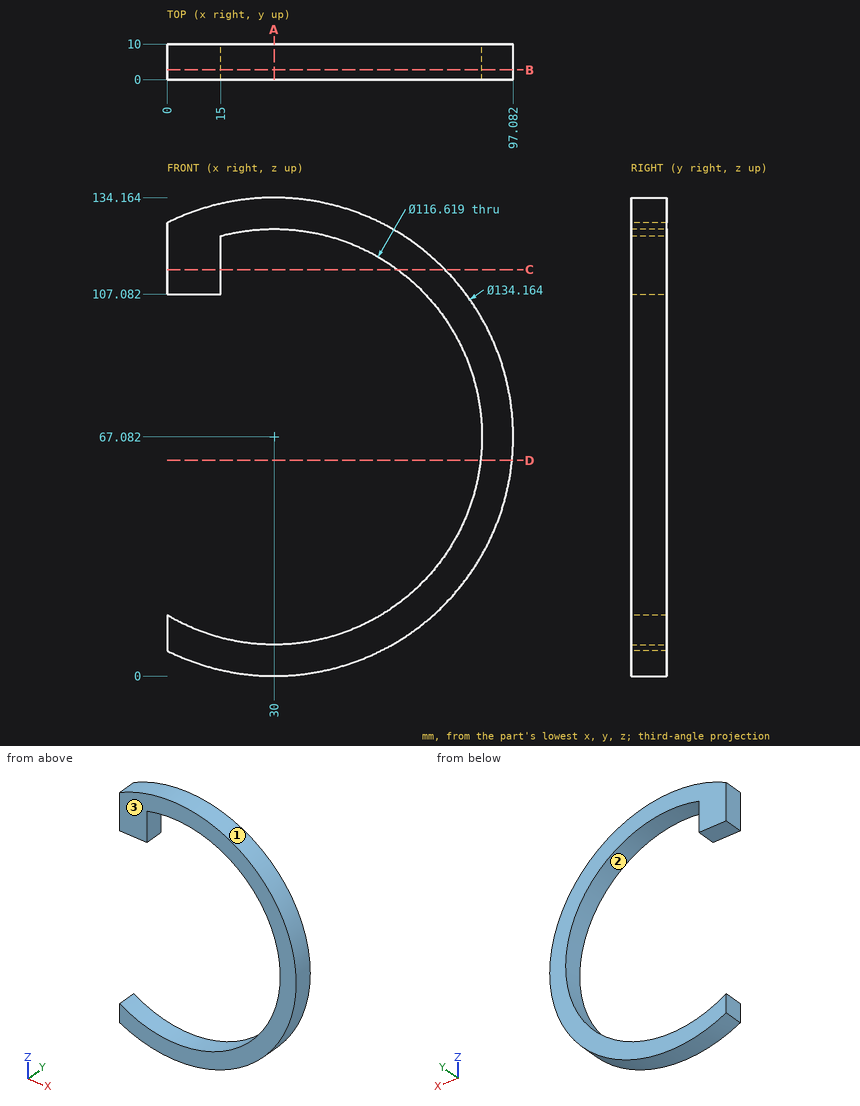
The drawing under review shows one solid part. Ordinate dimensions are in mm from its lowest x, y, z. Give positions to 0.01 mm unless a question says otherwise; leave off trailing zeros. Order: outer loops, then holes, each group sorted by start corner. A loop starts at its lowest first (then second) coordinate and runs counter-clockwise, first axis right, second up. Notation, with made-up numbers: (-2.5, -18.75) - (55.5, -18.75) arc R12 cw to (55.5, -1.75) - close; hole circle Ø2 at (-26, 11.25). An arc over 180 degrees is marked (long way). Answer as a JSON object with one key per item and string values. Group by question number.
Item 1: Draft analysis for pull direction X (two halves, no side actions). For the marked faces 1, 2 and 3, state which applies: pulls with the +X half, pulls with the -X half, needs draft (parallel to the pull), parting line crosses it, or undercut.
Item 2: Take a section at D-D on z = 60.5. Give the boundary of the cut face in (x, y).
Item 3: Clearance check with flat-ended pins moving along their axes: pin 1 Ø2 at (x, y) = (38, 7.5) entering from +Z; pin 2 Ø3 at (x, y) = (74.5, 3) entering from +Z; pin 3 Ø1.5 at (y, z) = (6.5, 76) entering from -X. State where each tip first meets the part, or that it passes through.
Item 4: Take a section at B-B on y = 2.75. Give the boundary of the cut face in (x, z), and give its area (3 significant figures).
Item 5: Take a section at C-C on z = 114. Give the boundary of the cut face in (x, y).
Item 6: Take a section at A-A on x = 30. Give the boundary of the cut face in (y, z), and give its area (3 significant figures).
Item 7: Wall thickness on line 1 along Z through (x, y) = (30, 7.25); line 2 along Z through (x, y) = (81.5, 0.5); line 3 along X through (y, z) = (5, 117.5): over which ranges is each line inside the solid? List them lowest first.
Reported:
{
 "1": {"face 1": "parting line crosses it", "face 2": "undercut", "face 3": "needs draft"},
 "2": {"outline": "(87.94, 0) - (96.76, 0) - (96.76, 10) - (87.94, 10) - close"},
 "3": {"pin 1": "z = 133.8", "pin 2": "z = 118.57", "pin 3": "x = 87.5"},
 "4": {"outline": "(0, 7.08) arc R67.08 ccw (long way) to (0, 127.08) - (0, 107.08) - (15, 107.08) - (15, 123.43) arc R58.31 cw (long way) to (0, 17.08) - close", "area": "2,480 mm^2"},
 "5": {"outline": "(0, 0) - (15, 0) - (15, 10) - (0, 10) - close; (64.62, 0) - (77.94, 0) - (77.94, 10) - (64.62, 10) - close"},
 "6": {"outline": "(0, 0) - (10, 0) - (10, 8.77) - (0, 8.77) - close; (0, 125.39) - (10, 125.39) - (10, 134.16) - (0, 134.16) - close", "area": "175 mm^2"},
 "7": {"line 1": "0 to 8.77, 125.39 to 134.16", "line 2": "24.1 to 39.74, 94.43 to 110.07", "line 3": "0 to 15, 59.29 to 74.25"}
}
